```python
from build123d import *

# Parameters (mm, degrees)
SKETCH1_R           = 7
BOSS_EXTRUDE1_DEPTH = 44
SKETCH2_R           = 5.5
CUT_EXTRUDE1_DEPTH  = 99.636339936
CUT_EXTRUDE2_START  = -19
CUT_EXTRUDE2_DEPTH  = 19
CUT_EXTRUDE3_DEPTH  = 24


with BuildPart() as part:
    # Sketch1 → Boss-Extrude1 (new body)
    with BuildSketch(Plane.XY):
        with BuildLine():
            ThreePointArc((-40.404910175, -1.633500031), (-37.139674394, -2.846913799), (-35.459271434, -5.898205914))
            ThreePointArc((-35.459271434, -5.898205914), (-33.122441231, -13.749172092), (-28.683469034, -20.633500031))
            Line((-28.683469034, -20.633500031), (-22.980449087, -20.633500031))
            Line((-22.980449087, -20.633500031), (6.019550913, 13.366499969))
            Line((6.019550913, 13.366499969), (6.019550913, 32.366499969))
            Line((6.019550913, 32.366499969), (1.019550913, 37.366499969))
            Line((1.019550913, 37.366499969), (-22.980449087, 37.366499969))
            ThreePointArc((-22.980449087, 37.366499969), (-28.648710625, 28.077944899), (-39.256864445, 25.654410975))
            Line((-39.256864445, 25.654410975), (-65.980449087, 30.366499969))
            Line((-65.980449087, 30.366499969), (-72.980449087, 30.366499969))
            Line((-72.980449087, 30.366499969), (-79.980449087, 23.366499969))
            Line((-79.980449087, 23.366499969), (-79.980449087, 5.366499969))
            Line((-79.980449087, 5.366499969), (-72.980449087, -1.633500031))
            Line((-72.980449087, -1.633500031), (-40.404910175, -1.633500031))
        make_face()
        with Locations((-65.980449087, 12.366499969)):
            Circle(SKETCH1_R, mode=Mode.SUBTRACT)
    extrude(amount=BOSS_EXTRUDE1_DEPTH)

    # Sketch2 → Cut-Extrude1 (cut, through all)
    with BuildSketch(Plane.XY.offset(44)):
        with Locations((-7.980449087, 23.366499969)):
            Circle(SKETCH2_R)
    extrude(amount=-CUT_EXTRUDE1_DEPTH, mode=Mode.SUBTRACT)

    # Sketch3 → Cut-Extrude2 (cut)
    with BuildSketch(Plane.XY.offset(44).offset(CUT_EXTRUDE2_START)):
        Polygon((-45.980449087, 26.839960355), (-45.980449087, -1.633500031), (-72.980449087, -1.633500031), (-79.980449087, 5.366499969), (-79.980449087, 23.366499969), (-72.980449087, 30.366499969), (-65.980449087, 30.366499969), align=None)
        with BuildLine():
            Line((-40.404910175, -1.633500031), (-6.774566734, -1.633500031))
            Line((-6.774566734, -1.633500031), (-22.980449087, -20.633500031))
            Line((-22.980449087, -20.633500031), (-28.683469034, -20.633500031))
            ThreePointArc((-28.683469034, -20.633500031), (-33.122441231, -13.749172092), (-35.459271434, -5.898205914))
            ThreePointArc((-35.459271434, -5.898205914), (-37.139674394, -2.846913799), (-40.404910175, -1.633500031))
        make_face()
    extrude(amount=CUT_EXTRUDE2_DEPTH, mode=Mode.SUBTRACT)

    # Sketch7 → Cut-Extrude3 (cut)
    with BuildSketch(Plane(origin=(0, 0, 12), x_dir=(-1, 0, 0), z_dir=(0, 0, -1))):
        with BuildLine():
            Line((-6.019550913, 13.366499969), (4.215743204, 1.366499969))
            ThreePointArc((4.215743204, 1.366499969), (21.210918642, 10.417084234), (32.200340902, 26.227892629))
            ThreePointArc((32.200340902, 26.227892629), (26.041094158, 30.514775107), (22.980449087, 37.366499969))
            Line((22.980449087, 37.366499969), (-1.019550913, 37.366499969))
            Line((-1.019550913, 37.366499969), (-6.019550913, 32.366499969))
            Line((-6.019550913, 32.366499969), (-6.019550913, 13.366499969))
        make_face()
    extrude(amount=-CUT_EXTRUDE3_DEPTH, mode=Mode.SUBTRACT)


solid = part.part
```
Input: part model. Units: mm. Frame: model coordinates. A direction names the side the tool comes from. Coordinates: 2 decimals unless noted, no trailing zeros. Order: outer loops, then holes, each group sorted by start corner. A loop starts at its lowest first (then second) coordinate and runs counter-clockwise, first axis right, second up. Notation, with made-up numbers: (60.25, 71.5) - (76.25, 71.5) arc R15 cw to (76.25, 84.5) - close; hole circle Ø5 at (-4, -38.75). An arc over 180 degrees is marked (long way). Put each result on its own line as item: value.
1. Line query: line 1 along Z through (x, y) = (-20.5, 14); line 2 along Z through (x, y) = (-72.5, 5); line 3 along X through (y, z) = (8, 24). Output: solid intervals per line, ascending.
Report:
line 1: z = 0 to 12, 36 to 44
line 2: z = 0 to 25
line 3: x = -79.98 to -71.45, -60.51 to -18.22
2. Cut plane D-D on x = -22. Return the cut outline in (y, z).
Report:
outline: (-19.48, 0) - (37.37, 0) - (37.37, 12) - (11.14, 12) - (11.14, 36) - (37.37, 36) - (37.37, 44) - (-1.63, 44) - (-1.63, 25) - (-19.48, 25) - close
3. Cut plane A-A on z = 17. Return the cut outline in (x, y).
Report:
outline: (-79.98, 5.37) - (-72.98, -1.63) - (-40.4, -1.63) arc R5 cw to (-35.46, -5.9) arc R29 ccw to (-28.68, -20.63) - (-22.98, -20.63) - (-4.22, 1.37) arc R41 cw to (-32.2, 26.23) arc R14 cw to (-39.26, 25.65) - (-65.98, 30.37) - (-72.98, 30.37) - (-79.98, 23.37) - close; hole circle Ø14 at (-65.98, 12.37)
4. Cut plane B-B on x = -0.5. Return the cut outline in (y, z), then the cut area to 3 significant figures.
Report:
outline: (5.72, 0) - (37.37, 0) - (37.37, 12) - (5.72, 12) - close; (5.72, 36) - (37.37, 36) - (37.37, 44) - (5.72, 44) - close
area: 633 mm2
5. Draft query along Y for faces 1 (the face through (-49.462, 27.454, 16.803)), 2 (the face through (-45.98, 13, 34)), 3 (the face through (-72.974, 12.674, 12.325)). Return one class per face: pulls with the +Y half, pulls with the -Y half, needs draft (parallel to the pull), parting line crosses it, or undercut.
Report:
face 1: pulls with the +Y half
face 2: needs draft
face 3: undercut
6. Reachability of faces 4 (the face through (6.02, 23, 40)), 5 (the face through (-59, 15, 25)), 6 (the face through (-21.01, 10.24, 23.83)) from +Z, -Z, +X, -X, +Y, -Y: full face, straight path, thin tool, end or side. Return the list, or none.
Report:
face 4: +Z, -Z, +X, +Y, -Y
face 5: +Z, -X, +Y, -Y
face 6: +X, +Y
7. Contact query for flat-ended pins moving along their axis: pin 1 Ø5 at (x, z) = (-41, 10.5) entering from -Y; pin 2 Ø10 at (x, z) = (-42.5, 27.5) entering from +Y; pin 3 Ø9.5 at (x, y) = (-22.5, -13) entering from +Z. Output: stop coordinate, or through.
Report:
pin 1: stops at y = -2.01
pin 2: stops at y = 26.99
pin 3: stops at z = 25
8. Cut plane C-C on z = 9.5. Return the cut outline in (x, y), then the cut area to 3 significant figures.
Report:
outline: (-79.98, 5.37) - (-72.98, -1.63) - (-40.4, -1.63) arc R5 cw to (-35.46, -5.9) arc R29 ccw to (-28.68, -20.63) - (-22.98, -20.63) - (6.02, 13.37) - (6.02, 32.37) - (1.02, 37.37) - (-22.98, 37.37) arc R14 cw to (-39.26, 25.65) - (-65.98, 30.37) - (-72.98, 30.37) - (-79.98, 23.37) - close; hole circle Ø14 at (-65.98, 12.37); hole circle Ø11 at (-7.98, 23.37)
area: 2,800 mm2
